Verification items for the finished model (mm, model axes). A direction names the side the tool comes from. Round coordinates to 2 decimals unless told otherwise and drop trailing zeros. Order: outer loops, then holes, each group sorted by start corner. A loop starts at its lowest first (then second) coordinate and runs counter-clockwise, first axis right, second up. Notation, with made-up numbers: M 44,39 L 75,39 A35 cw 75,76 Z; hole C 65.25,54 d1. An arc over 180 degrees is marked long. Write item = value, one per line. Start each with the question number.
from build123d import *

# Parameters (mm, degrees)
SKETCH1_R           = 12.8
BOSS_EXTRUDE1_DEPTH = 20.1
SKETCH2_OUTSIDE_W   = 35.882
SKETCH2_OUTSIDE_H   = 35.882
SKETCH2_OUTSIDE_R   = 4.5
CUT_EXTRUDE1_DEPTH  = 6.5
CHAMFER1_SIZE       = 0.5
SKETCH3_R           = 3
CUT_EXTRUDE2_DEPTH  = 10
SKETCH4_OUTSIDE_W   = 35.882
SKETCH4_OUTSIDE_H   = 35.882
SKETCH4_OUTSIDE_W_2 = 13.6
SKETCH4_OUTSIDE_H_2 = 15.5
CUT_EXTRUDE3_DEPTH  = 13.6
SKETCH5_R           = 4.8
CUT_EXTRUDE4_DEPTH  = 13.5


with BuildPart() as part:
    # Sketch1 → Boss-Extrude1 (new body)
    with BuildSketch(Plane.XY):
        with Locations(Location((0, 0, 0), (0, 0, 180))):
            Circle(SKETCH1_R)
    extrude(amount=BOSS_EXTRUDE1_DEPTH)

    # Sketch2 outside → Cut-Extrude1 (cut)
    with BuildSketch(Plane.XY.offset(20.1)):
        Rectangle(SKETCH2_OUTSIDE_W, SKETCH2_OUTSIDE_H)
        Circle(SKETCH2_OUTSIDE_R, mode=Mode.SUBTRACT)
    extrude(amount=-CUT_EXTRUDE1_DEPTH, mode=Mode.SUBTRACT)

    # Chamfer1
    chamfer1_edges = [part.edges().sort_by_distance(p)[0] for p in [
        (-4.5, 0, 20.1),
    ]]
    chamfer(chamfer1_edges, length=CHAMFER1_SIZE)

    # Sketch3 → Cut-Extrude2 (cut)
    with BuildSketch(Plane.XY.offset(20.1)):
        Circle(SKETCH3_R)
    extrude(amount=-CUT_EXTRUDE2_DEPTH, mode=Mode.SUBTRACT)

    # Sketch4 outside → Cut-Extrude3 (cut)
    with BuildSketch(Plane.XY.offset(13.6)):
        Rectangle(SKETCH4_OUTSIDE_W, SKETCH4_OUTSIDE_H)
        with Locations((0, 2.25)):
            Rectangle(SKETCH4_OUTSIDE_W_2, SKETCH4_OUTSIDE_H_2, mode=Mode.SUBTRACT)
    extrude(amount=-CUT_EXTRUDE3_DEPTH, mode=Mode.SUBTRACT)

    # Sketch5 → Cut-Extrude4 (cut)
    with BuildSketch(Plane(origin=(0, 10, 0), x_dir=(1, 0, 0), z_dir=(0, 1, 0))):
        with Locations(Location((0, -6.8, 0), (0, 0, 270))):
            Circle(SKETCH5_R)
    extrude(amount=-CUT_EXTRUDE4_DEPTH, mode=Mode.SUBTRACT)


solid = part.part
1) Access from +Z, -Z, +X, -X, +Y, -Y to the whole of each face (thin tool, end or side, straight path). Record for faces 4 (the flat face through (0, -3.5, 7)), 5 (the flat face through (0, 2, 0)), 6 (the cylindrical face through (-3, 0, 15)).
2) Cross-section at C-C, the plane z = 4. Enter the section's corners in (x, y).
3) Release check for a two-part mould opening along X. For faces 1 (the cylindrical face through (0, 3, 2)), 2 (the flat face through (-6.8, 2, 7)), 3 (the flat face through (0, -5.5, 7)) record: pulls with the +X half, pulls with the -X half, needs draft (parallel to the pull), parting line crosses it, or undercut.
4) Scan lines: probe 1 along X at (y, z) = (5.5, 6.8); probe 2 along Y at (x, z) = (0, 14.5); probe 3 along Z at (x, y) = (5.25, 5.25). Record each from-to range of solid material in increasing order.
5) Cross-section at A-A, the plane x = 0. Enter the section's corners in (y, z).
6) Cross-section at D-D, the plane y = 0. Enter the section's corners in (x, z), then the cut area to 3 significant figures.
7) Cross-section at B-B, the plane y = 5.5. Enter the section's corners in (x, z), then the cut area to 3 significant figures.
8) Gauge pin test, flat ends, axial feed: P1, Ø3, axis at x = 1.5, z = 6.5, coming from the +Y side; P2, Ø4, axis at x = -0.5, y = 0.5, coming from the +Z side. Record the tip position at first contact, or that the pin passes through.
Geometry results:
q1.face_4 = +Y
q1.face_5 = -Z, +X, -X, +Y, -Y
q1.face_6 = +Z
q2.outline = M -6.8,-5.5 L 6.8,-5.5 L 6.8,10 L 3.9,10 L 3.9,-3.5 L -3.9,-3.5 L -3.9,10 L -6.8,10 Z
q3.face_1 = undercut
q3.face_2 = pulls with the -X half
q3.face_3 = needs draft
q4.probe_1 = -6.8 to -4.8, 4.8 to 6.8
q4.probe_2 = -4.5 to -3, 3 to 4.5
q4.probe_3 = 0 to 13.6
q5.outline = M -5.5,0 L 10,0 L 10,2 L -3.5,2 L -3.5,11.6 L -3,11.6 L -3,20.1 L -4,20.1 L -4.5,19.6 L -4.5,13.6 L -5.5,13.6 Z; M 3,11.6 L 10,11.6 L 10,13.6 L 4.5,13.6 L 4.5,19.6 L 4,20.1 L 3,20.1 Z
q6.outline = M -6.8,0 L 6.8,0 L 6.8,13.6 L 4.5,13.6 L 4.5,19.6 L 4,20.1 L 3,20.1 L 3,10.55 A4.8 cw long -3,10.55 L -3,20.1 L -4,20.1 L -4.5,19.6 L -4.5,13.6 L -6.8,13.6 Z
q6.area = 118 mm^2
q7.outline = M -6.8,0 L 6.8,0 L 6.8,13.6 L -6.8,13.6 Z; hole C 0,6.8 d9.6
q7.area = 113 mm^2
q8.P1 = -3.5
q8.P2 = 2.7
